Job drawing, mm, ordinate dimensions from the low corner. One solid piece. A direction names the side the tool comes from. Round coordinates to 2 decimals unless told otherwise and drop trailing zeros. Loops run counter-clockwise (first coordinate to the right, second up) from the corner with the lowest first, then second, coordinate; pieces in that order, holes last. Notation, with made-up numbers: M -11.5,61 L 18.5,61 A25 cw 18.5,96 Z; hole C -27,84.5 d6. An arc over 180 degrees is marked long. One line per item, written item: value.
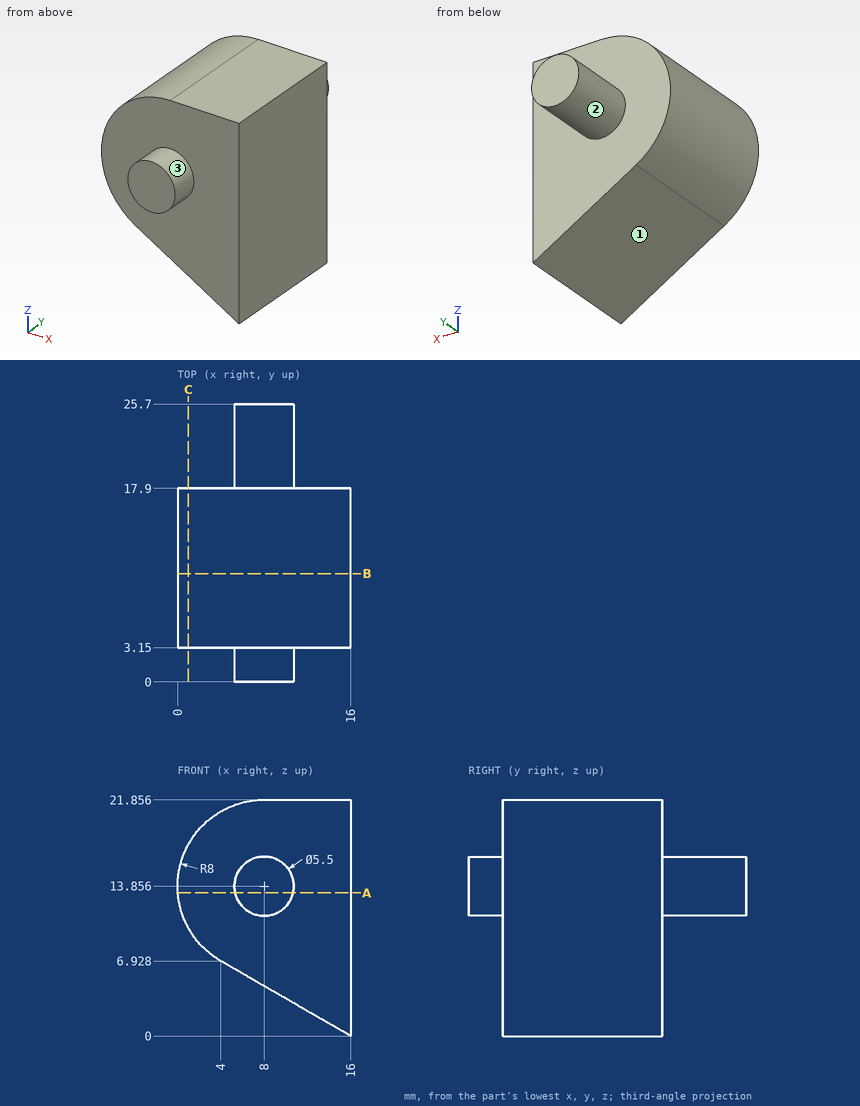
Item 1: Slice it at A-A, the plane z = 13.25. Give the cut face in (x, y), and give its area (3 significant figures).
Check values:
outline: M 0.02,3.15 L 5.32,3.15 L 5.32,0 L 10.68,0 L 10.68,3.15 L 16,3.15 L 16,17.9 L 10.68,17.9 L 10.68,25.7 L 5.32,25.7 L 5.32,17.9 L 0.02,17.9 Z
area: 294 mm2
Item 2: Wall check: line 1 along Y through (x, z) = (13.25, 15.5); line 2 along Z through (x, y) = (10.75, 3.5) (1 decimal); line 3 along X through (y, z) = (3.5, 13.25). Give the ranges that are in metal, low to high.
Check values:
line 1: y = 3.15 to 17.9
line 2: z = 3 to 21.9
line 3: x = 0.02 to 16
Item 3: Slice it at C-C, the plane x = 1. Give the cut face in (y, z).
Check values:
outline: M 3.15,9.98 L 17.9,9.98 L 17.9,17.73 L 3.15,17.73 Z
Item 4: Slice it at B-B, the plane y = 10. Give the cut face in (x, z), and give its area (3 significant figures).
Check values:
outline: M 4,6.93 L 16,0 L 16,21.86 L 8,21.86 A8 ccw Z
area: 259 mm2
Item 5: Drop flat-ended pins along their axis: P1, Ø3, axis at x = 11.5, z = 6, coming from the -Y side; P2, Ø5, axis at x = 6, y = 20, coming from the -Z side; P3, Ø5, axis at x = 8, z = 11, coming from the -Y side; P4, Ø6, axis at x = 2, z = 8, coming from the +Y side. Give the stop position or say it passes through.
Check values:
P1: stops at y = 3.15
P2: stops at z = 4.99
P3: stops at y = 0
P4: stops at y = 17.9
Item 6: Which spindle directions (+Z, -Z, +X, -X, +Y, -Y) get a long thin tool onto all of the face, cutting with end or side? Do the marked faces 1, 2 and 3. Say none if no direction does.
Check values:
face 1: -Z, -X, +Y, -Y
face 2: +Y
face 3: -Y
